```python
from build123d import *

# Parameters (mm, degrees)
SKETCH1_R           = 10.5
BOSS_EXTRUDE1_DEPTH = 4.5
SKETCH2_R           = 15
BOSS_EXTRUDE2_DEPTH = 10
SKETCH3_R           = 10
BOSS_EXTRUDE3_DEPTH = 25
SKETCH4_R           = 7.5
BOSS_EXTRUDE4_DEPTH = 8
SKETCH5_R           = 5.5
BOSS_EXTRUDE5_DEPTH = 3
CHAMFER1_SIZE       = 1
CHAMFER1_SIZE2      = 1.732050808


with BuildPart() as part:
    # Sketch1 → Boss-Extrude1 (new body)
    with BuildSketch(Plane(origin=(0, 0, 0), x_dir=(1, 0, 0), z_dir=(0, 1, 0))):
        with Locations(Location((0, 0, 0), (0, 0, 270))):
            Circle(SKETCH1_R)
    extrude(amount=BOSS_EXTRUDE1_DEPTH)

    # Sketch2 → Boss-Extrude2 (add)
    with BuildSketch(Plane(origin=(0, 4.5, 0), x_dir=(1, 0, 0), z_dir=(0, 1, 0))):
        with Locations(Location((0, 0, 0), (0, 0, 270))):
            Circle(SKETCH2_R)
    extrude(amount=BOSS_EXTRUDE2_DEPTH)

    # Sketch3 → Boss-Extrude3 (add)
    with BuildSketch(Plane(origin=(0, 14.5, 0), x_dir=(1, 0, 0), z_dir=(0, 1, 0))):
        with Locations(Location((0, 0, 0), (0, 0, 270))):
            Circle(SKETCH3_R)
    extrude(amount=BOSS_EXTRUDE3_DEPTH)

    # Sketch4 → Boss-Extrude4 (add)
    with BuildSketch(Plane(origin=(0, 39.5, 0), x_dir=(1, 0, 0), z_dir=(0, 1, 0))):
        with Locations(Location((0, 0, 0), (0, 0, 270))):
            Circle(SKETCH4_R)
    extrude(amount=BOSS_EXTRUDE4_DEPTH)

    # Sketch5 → Boss-Extrude5 (add)
    with BuildSketch(Plane(origin=(0, 47.5, 0), x_dir=(1, 0, 0), z_dir=(0, 1, 0))):
        with Locations(Location((0, 0, 0), (0, 0, 270))):
            Circle(SKETCH5_R)
    extrude(amount=BOSS_EXTRUDE5_DEPTH)

    # Chamfer1
    chamfer1_edges = [part.edges().sort_by_distance(p)[0] for p in [
        (0, 50.5, -5.5),
    ]]
    chamfer1_side = [part.faces().sort_by_distance(p)[0] for p in [
        (0, 49, -5.5),
    ]]
    chamfer(chamfer1_edges, length=CHAMFER1_SIZE, length2=CHAMFER1_SIZE2, reference=chamfer1_side[0])


solid = part.part
```
The listing builds one solid part. Answer for the finished solid, in the listing's coordinates (mm). A direction names the side the tool comes from. Give positions to 0.01 mm unless a question says otherwise; leave off trailing zeros. Order: outer loops, then holes, each group sorted by start corner. A loop starts at its lowest first (then second) coordinate and runs counter-clockwise, first axis right, second up. Notation, with made-up numbers: (-2.75, 82.25) - (43.25, 82.25) arc R22 cw to (43.25, 119.25) - close; hole circle Ø1 at (0, 17). An arc over 180 degrees is marked (long way). Use one line per item in the form item = value. Start each with the question number.
(1) For faces 1 (the flat face through (0, 0, 0)), 2 (the cylindrical face through (3.2, 2.2, 10)), 3 (the cylindrical face through (0.33, 43.444, -7.493)), determine the directions among +Z, -Z, +X, -X, +Y, -Y from which every point of the face is accessible in a straight line to the end or side of a thin tool.
(2) Flat-ended cylindrical pins translate along their axes: pin 1 Ø4 at (x, y) = (9, 27) entering from -Z; pin 2 Ø4 at (y, z) = (38.5, -1) entering from -X; pin 3 Ø6 at (y, z) = (12.5, 8.5) entering from -X. Find the tip coordinate at first contact, or state that the pin passes through.
(3) A cutting plane is placed at D-D, the plane x = 6.75. Write down the section's boundary in (y, z).
(4) A cutting plane is placed at C-C, the plane y = 12.5. Write down the section's boundary in (x, z).
(5) A cutting plane is placed at B-B, the plane z = 0. Write down the section's boundary in (x, y), then the cut area to 3 significant figures.
(6) A cutting plane is placed at A-A, the plane x = 0. Write down the section's boundary in (y, z), then the cut area to 3 significant figures.
(7) Consider line 1 (Y direction, x = -7.25, z = 12.75); line 2 (Y direction, x = 5, z = 4.5); line 3 (Z direction, x = -3.5, y = 13.5). Determine where each line is inside the solid, lowest interval first. Write a range as from..to.
Ans:
q1.face_1 = +Z, -Z, +X, -X, -Y
q1.face_2 = -Y
q1.face_3 = +Y
q2.pin_1 = -7.14
q2.pin_2 = -10
q2.pin_3 = -13.96
q3.outline = (0, -8.04) - (4.5, -8.04) - (4.5, -13.4) - (14.5, -13.4) - (14.5, -7.38) - (39.5, -7.38) - (39.5, -3.27) - (47.5, -3.27) - (47.5, 3.27) - (39.5, 3.27) - (39.5, 7.38) - (14.5, 7.38) - (14.5, 13.4) - (4.5, 13.4) - (4.5, 8.04) - (0, 8.04) - close
q4.outline = circle Ø30 at (0, 0)
q5.outline = (-15, 4.5) - (-10.5, 4.5) - (-10.5, 0) - (10.5, 0) - (10.5, 4.5) - (15, 4.5) - (15, 14.5) - (10, 14.5) - (10, 39.5) - (7.5, 39.5) - (7.5, 47.5) - (5.5, 47.5) - (5.5, 49.5) - (3.77, 50.5) - (-3.77, 50.5) - (-5.5, 49.5) - (-5.5, 47.5) - (-7.5, 47.5) - (-7.5, 39.5) - (-10, 39.5) - (-10, 14.5) - (-15, 14.5) - close
q5.area = 1,050 mm^2
q6.outline = (0, -10.5) - (4.5, -10.5) - (4.5, -15) - (14.5, -15) - (14.5, -10) - (39.5, -10) - (39.5, -7.5) - (47.5, -7.5) - (47.5, -5.5) - (49.5, -5.5) - (50.5, -3.77) - (50.5, 3.77) - (49.5, 5.5) - (47.5, 5.5) - (47.5, 7.5) - (39.5, 7.5) - (39.5, 10) - (14.5, 10) - (14.5, 15) - (4.5, 15) - (4.5, 10.5) - (0, 10.5) - close
q6.area = 1,050 mm^2
q7.line_1 = 4.5..14.5
q7.line_2 = 0..47.5
q7.line_3 = -14.59..14.59
